Design review of the part built by this model. Coordinates are the model's own, in mm. Face numbers are marked on the shaded views. A direction names the side the tool comes from. Round coordinates to 2 decimals unless told otherwise and drop trailing zeros. Loops run counter-clockwise (first coordinate to the right, second up) from the corner with the lowest first, then second, coordinate; pieces in that order, holes last. Notation, with made-up numbers: M 1,-7.5 L 33,-7.5 A20 ccw 33,5.5 Z; hole C 40.5,-1 d5. An arc over 180 degrees is marked long. One line per item, written item: value. Start each with the question number.
Item 1: Clearance check with flat-ended pins moving along their axes: pin 1 (1.5 mm diameter, centred on x = 6.5, z = 9, fed in from +Y); pin 2 (8 mm diameter, centred on y = 6.5, z = 6.5, fed in from +X); pin 3 (2 mm diameter, centred on x = 3.5, z = 9.5, fed in from +Y). State where each tip first meets the part, or that it passes through.
Item 2: For line 1 along X through (y, z) = (3, 15.25) (3 decimals); line 2 along Z through (x, y) = (-4.25, 0.5); line 3 along Y through (x, z) = (-2.3, 17), list the stretches that pass through material, from the lowest coordinate up.
Item 3: For the marked faces 4, 5, 6 and 7, list the 3-axis set-ups (+Z, -Z, +X, -X, +Y, -Y) from which the entire face can be reached by the end or side of a thin tool; tool diameter is ignored.
Item 4: We need section C-C (y = 3.75). State how many separate pieces and enclosed holes the cut face has, then the cut area to 3 significant figures.
Item 5: Mouldability with a two-part tool opening along X and no side actions: class the marked faces 1, 2 and 3 as released by +X, released by -X, zero draft, split by the parting line, or undercut.
Item 6: We need section A-A (z = 17). Write out the cut boundary in (x, y) (3 decimals), then the cut area to 3 significant figures.
Item 7: We need section B-B (z = 6.5). Write out the cut boundary in (x, y) (3 decimals).
Item 8: We need section D-D (x = -4). Write out the cut boundary in (y, z), then the cut area to 3 significant figures.
from build123d import *

# Parameters (mm, degrees)
SKETCH1_W               = 16.25
SKETCH1_H               = 16.25
SKETCH1_W_2             = 12.25
SKETCH1_H_2             = 12.25
BOSS_EXTRUDE1_DEPTH     = 5
FILLET1_R               = 5
SKETCH2_W               = 18.25
SKETCH2_H               = 18.25
BOSS_EXTRUDE2_DEPTH     = 2
FILLET2_R               = 7
BOSS_EXTRUDE3_DEPTH     = 20
CUT_EXTRUDE1_DEPTH      = 30.925428151
CUT_EXTRUDE1_DEPTH_BACK = 30.925428151
SKETCH5_R               = 1.6
SKETCH7_R               = 3
CUT_EXTRUDE2_DEPTH      = 5.5
CUT_EXTRUDE3_DEPTH      = 4
SKETCH9_W               = 3
SKETCH9_H               = 10.743898354
CUT_EXTRUDE4_DEPTH      = 34.096015703


with BuildPart() as part:
    # Sketch1 → Boss-Extrude1 (new body)
    with BuildSketch(Plane.XY):
        Rectangle(SKETCH1_W, SKETCH1_H)
        Rectangle(SKETCH1_W_2, SKETCH1_H_2, mode=Mode.SUBTRACT)
    extrude(amount=BOSS_EXTRUDE1_DEPTH)

    # Fillet1
    fillet1_edges = [part.edges().sort_by_distance(p)[0] for p in [
        (6.125, -6.125, 2.5),
        (6.125, 6.125, 2.5),
        (-6.125, 6.125, 2.5),
        (-6.125, -6.125, 2.5),
        (-8.125, 8.125, 2.5),
        (8.125, 8.125, 2.5),
        (8.125, -8.125, 2.5),
        (-8.125, -8.125, 2.5),
    ]]
    fillet(fillet1_edges, radius=FILLET1_R)

    # Sketch2 → Boss-Extrude2 (add)
    with BuildSketch(Plane.XY.offset(5)):
        Rectangle(SKETCH2_W, SKETCH2_H)
    extrude(amount=BOSS_EXTRUDE2_DEPTH)

    # Fillet2
    fillet2_edges = [part.edges().sort_by_distance(p)[0] for p in [
        (-9.125, 9.125, 6),
        (-9.125, -9.125, 6),
        (9.125, -9.125, 6),
        (9.125, 9.125, 6),
    ]]
    fillet(fillet2_edges, radius=FILLET2_R)

    # Sketch3 → Boss-Extrude3 (add)
    with BuildSketch(Plane.XY.offset(7)):
        with BuildLine():
            Line((1, 7.634788799), (1, 2.507987241))
            ThreePointArc((1, 2.507987241), (0, -2.7), (-1, 2.507987241))
            Line((-1, 2.507987241), (-1, 7.634788799))
            ThreePointArc((-1, 7.634788799), (0, -7.7), (1, 7.634788799))
        make_face()
    extrude(amount=BOSS_EXTRUDE3_DEPTH)

    # Sketch5 → Cut-Extrude1 (cut, two sides: drawn at the far end of the back side and taken through both)
    with BuildSketch(Plane(origin=(0, 0, 0), x_dir=(0, 0, -1), z_dir=(1, 0, 0)).offset(-CUT_EXTRUDE1_DEPTH_BACK)):
        with Locations((-17, 4.979474194)):
            Circle(SKETCH5_R)
    extrude(amount=CUT_EXTRUDE1_DEPTH + CUT_EXTRUDE1_DEPTH_BACK, mode=Mode.SUBTRACT)

    # Sketch7 → Cut-Extrude2 (cut)
    with BuildSketch(Plane(origin=(9.125, 0, 0), x_dir=(0, 0, -1), z_dir=(1, 0, 0))):
        with Locations((-17, 4.979474194)):
            Circle(SKETCH7_R)
    extrude(amount=-CUT_EXTRUDE2_DEPTH, mode=Mode.SUBTRACT)

    # Sketch8 → Cut-Extrude3 (cut)
    with BuildSketch(Plane.ZY.offset(7.7)):
        Polygon((13.420428331, 4.979474194), (15.210214166, 1.879474194), (18.789785834, 1.879474194), (20.579571669, 4.979474194), (18.789785834, 8.079474194), (15.210214166, 8.079474194), align=None)
    extrude(amount=-CUT_EXTRUDE3_DEPTH, mode=Mode.SUBTRACT)

    # Sketch9 → Cut-Extrude4 (cut, through all)
    with BuildSketch(Plane.ZY.offset(7.7)):
        with Locations((8.5, 5.371949177)):
            Rectangle(SKETCH9_W, SKETCH9_H)
    extrude(amount=-CUT_EXTRUDE4_DEPTH, mode=Mode.SUBTRACT)


solid = part.part
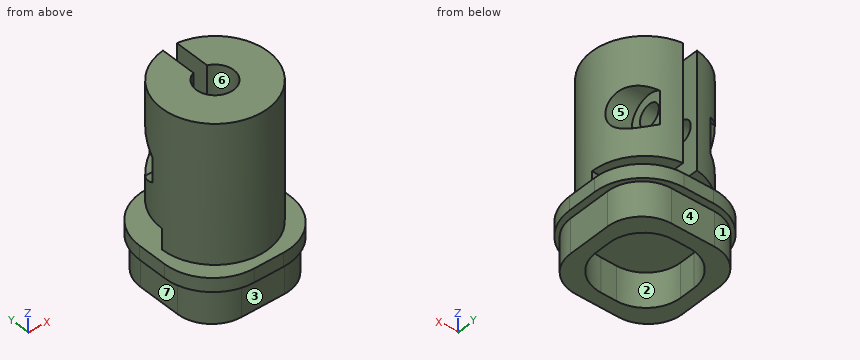
A:
1. pin 1: y = 0
1. pin 2: x = 9.11
1. pin 3: y = 7.24
2. line 1: -3.7 to -1, 1 to 3.625
2. line 2: 5 to 7, 10 to 27
2. line 3: -7.35 to -1.41, 1.41 to 3.38, 6.58 to 7.35
3. face 4: -Z, +X, -X, +Y
3. face 5: +X
3. face 6: +Z
3. face 7: -Z, -X, +Y, -Y
4. separate pieces: 5
4. enclosed holes: 0
4. area: 212 mm2
5. face 1: released by -X
5. face 2: undercut
5. face 3: zero draft
6. outline: M -7.467,1.879 A7.7 ccw long 7.441,1.979 L 3.625,1.979 L 3.625,3.379 L 1,3.379 L 1,2.508 A2.7 cw long -1,2.508 L -1,3.379 L -3.7,3.379 L -3.7,1.879 Z; M -3.7,6.579 L -1,6.579 L -1,7.635 A7.7 ccw -3.7,6.753 Z; M 1,6.579 L 3.625,6.579 L 3.625,6.793 A7.7 ccw 1,7.635 Z
6. area: 113 mm2
7. outline: M -9.125,-2.125 A7 ccw -2.125,-9.125 L 2.125,-9.125 A7 ccw 9.125,-2.125 L 9.125,2.125 A7 ccw 2.125,9.125 L -2.125,9.125 A7 ccw -9.125,2.125 Z
8. outline: M -8.87,5 L -8.05,5 L -8.05,0 L -5.22,0 L -5.22,5 L 5.22,5 L 5.22,0 L 8.05,0 L 8.05,5 L 8.87,5 L 8.87,7 L 0,7 L 0,10 L 6.58,10 L 6.58,14.34 L 4.98,13.42 L 1.88,15.21 L 1.88,18.79 L 4.98,20.58 L 6.58,19.66 L 6.58,27 L -6.58,27 L -6.58,7 L -8.87,7 Z
8. area: 281 mm2
